Geometry check sheet. Reference: drawing and pictorial views, mm from the part's lowest x, y, z. Round coordinates to 2 decimals unless told otherwise and drop trailing zeros. Order: outer loops, then holes, each group sorted by start corner. A loop starts at its lowest first (then second) coordinate and runs counter-clockwise, first axis right, second up.
(1) Go/stop test with a flat-tipped pin: pin 1 (11 mm diameter, centred on x = 229, y = 177.5, fed in from +Z). Record where the tip stops, or that it passes through.
(2) Sectioned sample at C-C (z = 1). Record the boundary of the cut face in (x, y).
(3) Material ranges on line 1 along Y through (x, z) = (25, 2); line 2 along X through (y, z) = (102, 5); line 3 along X through (y, z) = (175, 5.75), recorded low to high.
(4) Sectioned sample at B-B (x = 229). Record the boundary of the cut face in (y, z), plus the area to 3 significant figures.
(5) Sectioned sample at D-D (y = 114). Record the boundary of the cut face in (x, z).
(6) Sectioned sample at A-A (y = 177.5). Record the boundary of the cut face in (x, z).
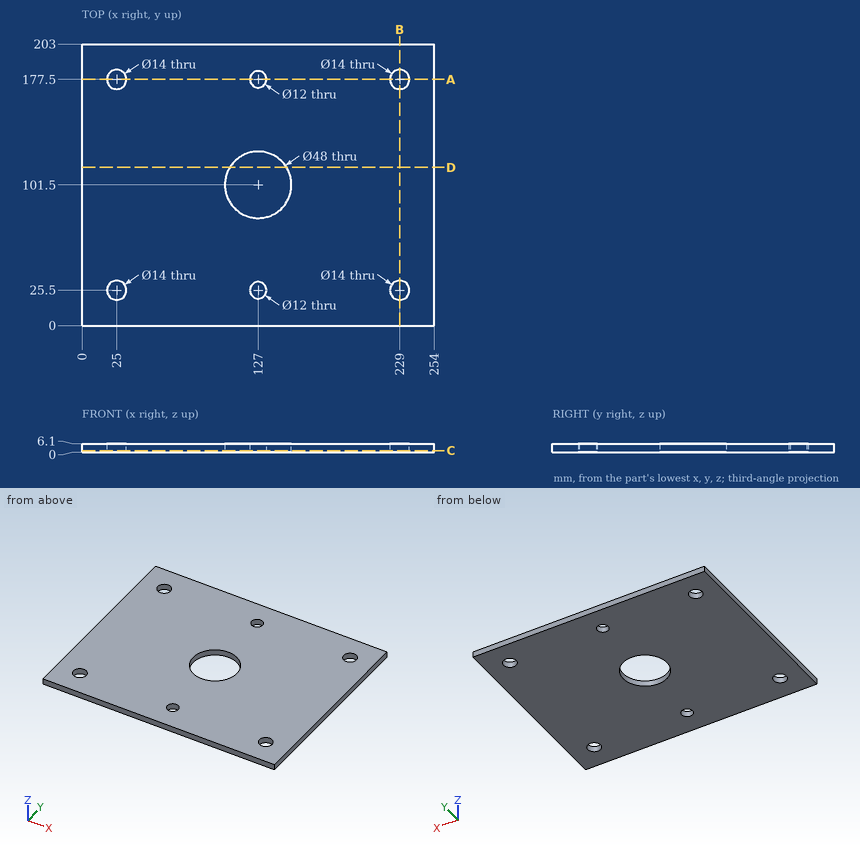
Answer below:
1. pin 1: passes through
2. outline: (0, 0) - (254, 0) - (254, 203) - (0, 203) - close; hole circle Ø14 at (25, 25.5); hole circle Ø14 at (25, 177.5); hole circle Ø48 at (127, 101.5); hole circle Ø12 at (127, 25.5); hole circle Ø12 at (127, 177.5); hole circle Ø14 at (229, 25.5); hole circle Ø14 at (229, 177.5)
3. line 1: y = 0 to 18.5, 32.5 to 170.5, 184.5 to 203
3. line 2: x = 0 to 103.01, 150.99 to 254
3. line 3: x = 0 to 18.46, 31.54 to 121.55, 132.45 to 222.46, 235.54 to 254
4. outline: (0, 0) - (18.5, 0) - (18.5, 6.1) - (0, 6.1) - close; (32.5, 0) - (170.5, 0) - (170.5, 6.1) - (32.5, 6.1) - close; (184.5, 0) - (203, 0) - (203, 6.1) - (184.5, 6.1) - close
4. area: 1,070 mm2
5. outline: (0, 0) - (106.51, 0) - (106.51, 6.1) - (0, 6.1) - close; (147.49, 0) - (254, 0) - (254, 6.1) - (147.49, 6.1) - close
6. outline: (0, 0) - (18, 0) - (18, 6.1) - (0, 6.1) - close; (32, 0) - (121, 0) - (121, 6.1) - (32, 6.1) - close; (133, 0) - (222, 0) - (222, 6.1) - (133, 6.1) - close; (236, 0) - (254, 0) - (254, 6.1) - (236, 6.1) - close
